Geometry: see drawing. Coordinates: mm, zero at the bounding-box minimum. Give positions to 0.01 mm unless a question says otherwise; leave off trailing zeros. Order: outer loops, then holes, each group sorted by start corner. A loop starts at its lowest first (then second) coordinate and runs counter-clockwise, first axis right, second up. Notation, with made-up numbers: (-6, 52.25) -> (33, 52.25) arc R18 ccw to (33, 68.25) -> close; hole circle Ø8 at (71.5, -27.5). An arc over 180 degrees is marked (long way). One line per item, written item: value. Start each with the question number.
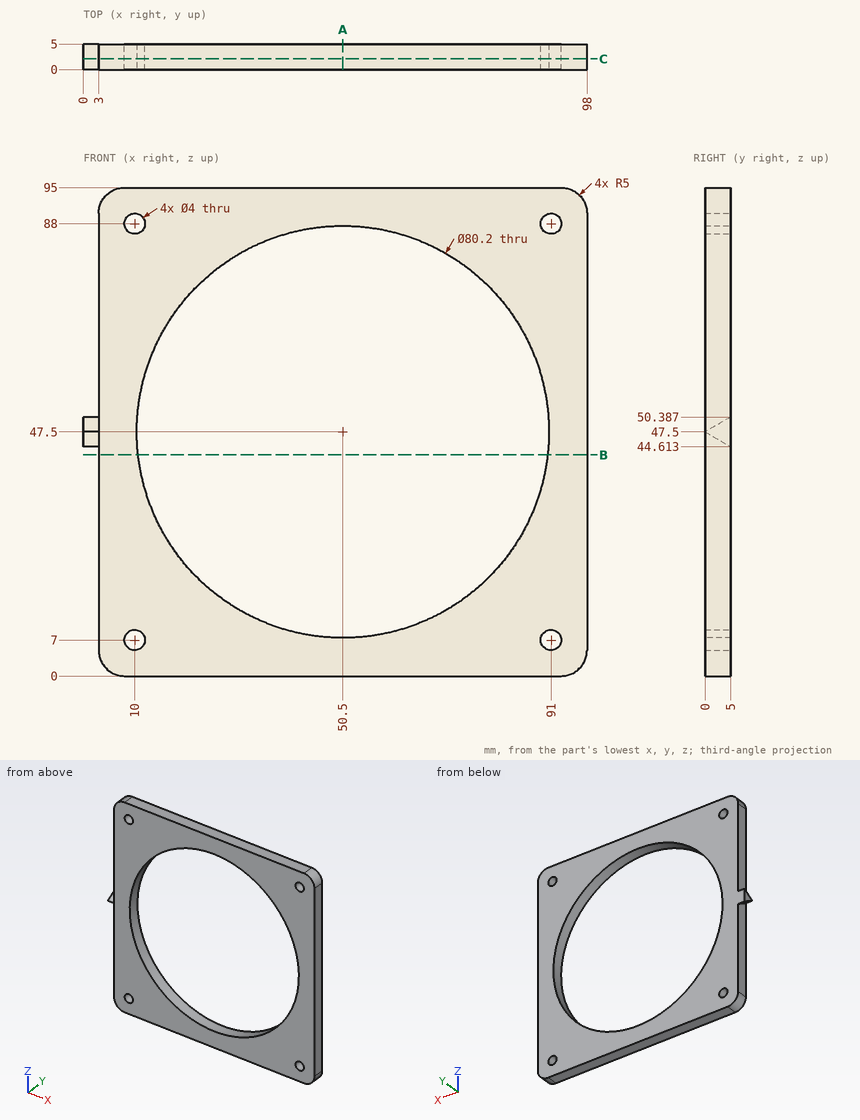
1. Cut plane C-C, the plane y = 2.1. Return loops of the section in (x, z), then the cut area to 3 significant figures.
2. Pin query (flat end, axial travel): P1, Ø2, axis at y = 1, z = 84, coming from the -X side. Return the tip coordinate at first contact, or that it passes through.
3. Material intervals for L1, parallel to X at y = 1.7, z = 7; L2, parallel to Z at x = 10, y = 3.1; L3, parallel to X at y = 3.85, z = 47.5, sorted ascending. Write a range as [from, to].
4. Cut plane A-A, the plane x = 50.5. Return loops of the section in (y, z).
5. Cut plane B-B, the plane z = 43. Return loops of the section in (x, y).
Answers follow:
1. outline: (0, 46.29) -> (3, 46.29) -> (3, 5) arc R5 ccw to (8, 0) -> (93, 0) arc R5 ccw to (98, 5) -> (98, 90) arc R5 ccw to (93, 95) -> (8, 95) arc R5 ccw to (3, 90) -> (3, 48.71) -> (0, 48.71) -> close; hole circle Ø4 at (10, 7); hole circle Ø4 at (10, 88); hole circle Ø80.2 at (50.5, 47.5); hole circle Ø4 at (91, 7); hole circle Ø4 at (91, 88)
1. area: 3,910 mm²
2. P1: stops at x = 3
3. L1: x = [3, 8], [12, 89], [93, 98]
3. L2: z = [0, 5], [9, 86], [90, 95]
3. L3: x = [0, 10.4], [90.6, 98]
4. outline: (0, 0) -> (5, 0) -> (5, 7.4) -> (0, 7.4) -> close; (0, 87.6) -> (5, 87.6) -> (5, 95) -> (0, 95) -> close
5. outline: (3, 0) -> (10.65, 0) -> (10.65, 5) -> (3, 5) -> close; (90.35, 0) -> (98, 0) -> (98, 5) -> (90.35, 5) -> close
